Geometry check sheet. Reference: the model listing, model coordinates, mm. Face numbers are marked on the shaded views. A direction names the side the tool comes from. Round coordinates to 2 decimals unless told otherwise and drop trailing zeros. Order: outer loops, then holes, each group sorted by start corner. A loop starts at its lowest first (then second) coordinate and runs counter-clockwise, first axis right, second up. Notation, with made-up numbers: (12, 11) - (32, 11) arc R29 cw to (32, 36) - close; hole circle Ø3 at (51.5, 48.25). An arc over 180 degrees is marked (long way). Return JSON: item names as keys, results as strings. Group by question number.
Q1. Sectioned sample at C-C, the plane x = -22. Record the cut outline in (y, z), then the cut area to 3 significant figures.
Q2. Sectioned sample at B-B, the plane y = -6. Record the cut outline in (x, z) (3 decimals).
Q3. Material ranges on line 1 along Z through (x, y) = (0, -8.5); line 2 along Z through (x, y) = (47, -27); line 3 along X through (y, z) = (-32.5, 45), recorded low to high.
Q4. Sectioned sample at D-D, the plane x = -60. Record the cut outline in (y, z), then the cut area to 3 significant figures.
Q5. Sectioned sample at A-A, the plane z = 28. Record the cut outline in (x, y), then the cut area to 3 significant figures.
Q6. Gauge pin test, flat ends, axial feed: pin 1 Ø3.5 at (y, z) = (19, 49.5) entering from +X; pin 2 Ø9 at (x, y) = (54, 31) entering from +Z; pin 3 Ø19 at (y, z) = (-14, 31) entering from -X; pin 4 Ø5 at (x, y) = (45.5, -0.5) entering from -Z. Record the tip position at first contact, or that the pin passes through.
Q7. Tool access check on the marked faces 1, 2 and 3. Record the directions out of +Z, -Z, +X, -X, +Y, -Y that give a thin tool (end or side, any length) a straight path to the whole face; none if there is none.
```python
from build123d import *

# Parameters (mm, degrees)
F0_W     = 146.05
F0_H     = 79.375
F1_DEPTH = 14.859
F3_DEPTH = 79.375
F4_DEPTH = 85.725
F6_DEPTH = 79.376
F8_DEPTH = 10.16


with BuildPart() as f1:
    # F0 (on Top) → F1 (new body)
    with BuildSketch(Plane.XY):
        Rectangle(F0_W, F0_H)
    extrude(amount=F1_DEPTH)

    # F2 (on face) → F3 (join)
    with BuildSketch(Plane.XZ.offset(39.6875)):
        with BuildLine():
            Line((-57.15, 14.859), (-15.875, 14.859))
            ThreePointArc((-15.875, 14.859), (-22.8952505992, 87.3018758988), (41.275, 52.959))
            ThreePointArc((41.275, 52.959), (34.3428758988, 30.0637494008), (15.875, 14.859))
            Line((15.875, 14.859), (57.15, 14.859))
            Line((57.15, 14.859), (57.15, 52.959))
            Line((57.15, 52.959), (45.72, 52.959))
            ThreePointArc((45.72, 52.959), (0, 98.679), (-45.72, 52.959))
            Line((-45.72, 52.959), (-57.15, 52.959))
            Line((-57.15, 52.959), (-57.15, 14.859))
        make_face()
    extrude(amount=-F3_DEPTH)

    # F2 (on face) → F4 (cut)
    with BuildSketch(Plane.XZ.offset(39.6875)):
        with BuildLine():
            Line((0, 14.859), (0, 11.684))
            ThreePointArc((0, 11.684), (8.0946934778, 12.4855326109), (15.875, 14.859))
            Line((15.875, 14.859), (0, 14.859))
        make_face()
        with BuildLine():
            ThreePointArc((-15.875, 14.859), (-8.0946934778, 12.4855326109), (0, 11.684))
            Line((0, 11.684), (0, 14.859))
            Line((0, 14.859), (-15.875, 14.859))
        make_face()
    extrude(amount=-F4_DEPTH, mode=Mode.SUBTRACT)

    # F5 (on face) → F6 (cut, through all)
    with BuildSketch(Plane.XZ.offset(39.6875)):
        with BuildLine():
            Line((57.15, 37.7415791154), (57.15, 41.5375120938))
            Line((57.15, 41.5375120938), (39.6632731757, 41.5375120938))
            ThreePointArc((39.6632731757, 41.5375120938), (39.0614634109, 39.6237946698), (38.3673784174, 37.7415791154))
            Line((38.3673784174, 37.7415791154), (57.15, 37.7415791154))
        make_face()
    extrude(amount=-F6_DEPTH, mode=Mode.SUBTRACT)

    # F7 (on face) → F8 (cut)
    with BuildSketch(Plane.XY.offset(52.959)):
        with BuildLine():
            Line((57.15, 17.8361811879), (57.15, 24.4548188121))
            ThreePointArc((57.15, 24.4548188121), (51.435, 27.7495), (45.72, 24.4548188121))
            Line((45.72, 24.4548188121), (45.72, 17.8361811879))
            ThreePointArc((45.72, 17.8361811879), (51.435, 14.5415), (57.15, 17.8361811879))
        make_face()
        with BuildLine():
            Line((57.15, -24.4548188121), (57.15, -17.8361811879))
            ThreePointArc((57.15, -17.8361811879), (51.435, -14.5415), (45.72, -17.8361811879))
            Line((45.72, -17.8361811879), (45.72, -24.4548188121))
            ThreePointArc((45.72, -24.4548188121), (51.435, -27.7495), (57.15, -24.4548188121))
        make_face()
    extrude(amount=-F8_DEPTH, mode=Mode.SUBTRACT)


solid = f1.part
```
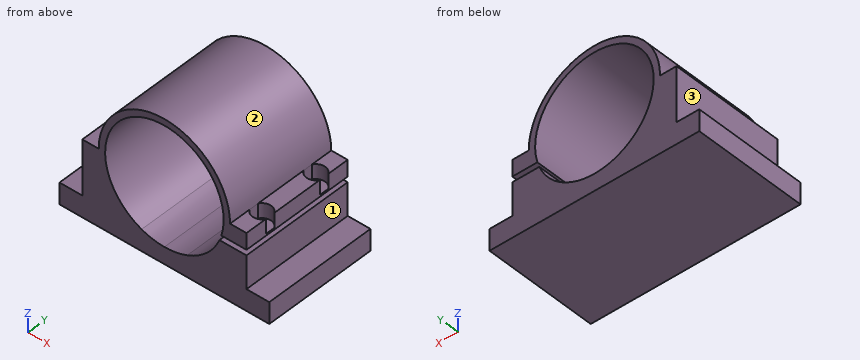
Reply:
{
 "1": {"outline": "(-39.69, 0) - (39.69, 0) - (39.69, 18.04) - (-39.69, 18.04) - close; (-39.69, 87.88) - (39.69, 87.88) - (39.69, 93.04) - (-39.69, 93.04) - close", "area": "1,840 mm^2"},
 "2": {"outline": "(-73.025, 0) - (73.025, 0) - (73.025, 14.859) - (57.15, 14.859) - (57.15, 37.742) - (38.367, 37.742) arc R41.275 cw (long way) to (39.663, 41.538) - (57.15, 41.538) - (57.15, 52.959) - (45.72, 52.959) arc R45.72 ccw to (-45.72, 52.959) - (-57.15, 52.959) - (-57.15, 14.859) - (-73.025, 14.859) - close"},
 "3": {"line 1": "0 to 11.68, 94.23 to 98.68", "line 2": "0 to 37.74, 41.54 to 52.96", "line 3": "-57.15 to -40.5, 40.5 to 57.15"},
 "4": {"outline": "(-39.69, 0) - (39.69, 0) - (39.69, 14.86) - (-39.69, 14.86) - close", "area": "1,180 mm^2"},
 "5": {"outline": "(-57.15, -39.69) - (-32.87, -39.69) - (-32.87, 39.69) - (-57.15, 39.69) - close; (32.87, -39.69) - (57.15, -39.69) - (57.15, 39.69) - (32.87, 39.69) - close", "area": "3,850 mm^2"},
 "6": {"pin 1": "x = 57.15", "pin 2": "z = 52.96", "pin 3": "x = -57.15", "pin 4": "z = 0"},
 "7": {"face 1": "+Z, +X, +Y, -Y", "face 2": "+Z, +Y, -Y", "face 3": "+Z, -X, +Y, -Y"}
}
